The listing builds one solid part. Answer for the finished solid, in the listing's coordinates (mm). Give positions to 0.01 mm unless a question says otherwise; leave off trailing zeros. Write each loop counter-clockwise with the first axis right and the second up, starting at its lowest first coordinate (ties: lowest second). Pieces come first, ordered by that corner, then holes. Notation, with made-up numbers: (-32, -35) -> (-1, -35) arc R26 cw to (-1, -12) -> close; hole circle Ø8 at (76.25, 51). An arc over 180 degrees is marked (long way). One line per question, with ' | ' between items.
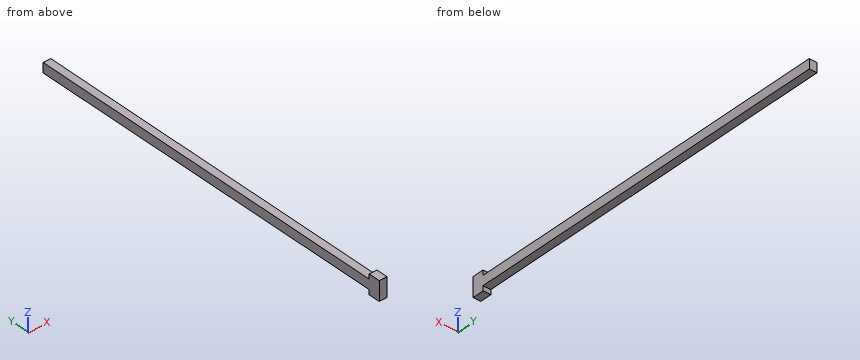
from build123d import *

# Parameters (mm, degrees)
SKETCH1_W             = 4
SKETCH1_H             = 2.501095517
BOSS_EXTRUDE1_DEPTH   = 6
SKETCH1_H_2           = 2.5
BOSS_EXTRUDE1_2_DEPTH = 6
SKETCH1_3_W           = 4
SKETCH1_3_H           = 5
BOSS_EXTRUDE2_DEPTH   = 200


with BuildPart() as part:
    # Sketch1 → Boss-Extrude1 (new body)
    with BuildSketch(Plane(origin=(0, 0, 0), x_dir=(1, 0, 0), z_dir=(0, 1, 0))):
        with Locations((0, -3.750547759)):
            Rectangle(SKETCH1_W, SKETCH1_H)
    extrude(amount=BOSS_EXTRUDE1_DEPTH)



with BuildPart() as body_2:
    # Sketch1 → Boss-Extrude1 2 (new body)
    with BuildSketch(Plane(origin=(0, 0, 0), x_dir=(1, 0, 0), z_dir=(0, 1, 0))):
        with Locations((0, 3.75)):
            Rectangle(SKETCH1_W, SKETCH1_H_2)
    extrude(amount=BOSS_EXTRUDE1_2_DEPTH)


with BuildPart() as part_1:
    add(part.part)

    add(body_2.part)  # Boss-Extrude2 merges body 2
    # Sketch1<3> → Boss-Extrude2 (add)
    with BuildSketch(Plane(origin=(0, 0, 0), x_dir=(1, 0, 0), z_dir=(0, 1, 0))):
        Rectangle(SKETCH1_3_W, SKETCH1_3_H)
    extrude(amount=BOSS_EXTRUDE2_DEPTH)


solid = part_1.part
Item 1: Find section A-A (x = -0.8). Write down the section's boundary in (y, z).
Answers below:
outline: (0, -5) -> (6, -5) -> (6, -2.5) -> (200, -2.5) -> (200, 2.5) -> (6, 2.5) -> (6, 5) -> (0, 5) -> close
Item 2: Find section B-B (y = 89). Write down the section's boundary in (x, z), then the cut area to 3 significant figures.
Answers below:
outline: (-2, -2.5) -> (2, -2.5) -> (2, 2.5) -> (-2, 2.5) -> close | area: 20.0 mm²
Item 3: Consider line 1 (Z direction, x = 0.3, y = 79.5); line 2 (Y direction, x = -0.3, z = -3.25). Determine where each line is inside the solid, lowest interval first. Write a range as [from, to].
Answers below:
line 1: [-2.5, 2.5] | line 2: [0, 6]
Item 4: Flat-ended cylindrical pins translate along their axes: pin 1 (1 mm diameter, centred on x = 0.5, y = 78, fed in from -Z); pin 2 (1.3 mm diameter, centred on x = -0.5, z = 4, fed in from +Y). Find the tip coordinate at first contact, or state that the pin passes through.
Answers below:
pin 1: z = -2.5 | pin 2: y = 6
